Model file for the job. Use its own axes, mm. Give positions to 0.01 mm unless a question says otherwise; leave off trailing zeros.
```python
from build123d import *

# Parameters (mm, degrees)
BOX_W     = 300
BOX_H     = 100
BOX_DEPTH = 140


with BuildPart() as cubo:
    # Box → Box (new body)
    with BuildSketch(Plane(origin=(50, -50, -70), x_dir=(1, 0, 0), z_dir=(0, 0, 1))):
        with Locations((150, 50)):
            Rectangle(BOX_W, BOX_H)
    extrude(amount=BOX_DEPTH)


with BuildPart() as loft001:
    # Sketch003 → Loft001 section 0
    with BuildSketch(Plane(origin=(-5, 0, 0), x_dir=(1, 0, 0), z_dir=(0, 0, 1))):
        Polygon((300, 0), (299.703, 0.018), (298.818, 0.072), (297.342, 0.183), (295.287, 0.363), (292.659, 0.621), (289.467, 0.957), (285.723, 1.368), (281.445, 1.851), (276.648, 2.403), (271.353, 3.027), (265.578, 3.732), (259.344, 4.509), (252.681, 5.364), (245.613, 6.288), (238.167, 7.281), (230.373, 8.337), (222.264, 9.45), (213.867, 10.611), (205.218, 11.811), (196.353, 13.038), (187.305, 14.286), (178.107, 15.534), (168.801, 16.767), (159.42, 17.97), (150, 19.119), (140.583, 20.193), (131.199, 21.174), (121.893, 22.038), (112.698, 22.761), (103.647, 23.322), (94.782, 23.703), (86.133, 23.886), (77.736, 23.856), (69.627, 23.607), (61.833, 23.127), (54.387, 22.419), (47.319, 21.486), (40.656, 20.34), (34.422, 18.996), (28.647, 17.472), (23.352, 15.798), (18.555, 13.998), (14.277, 12.105), (10.533, 10.155), (7.341, 8.184), (4.713, 6.246), (2.658, 4.41), (1.182, 2.745), (0.297, 1.281), (0, 0), (0.297, -1.17), (1.182, -2.301), (2.658, -3.432), (4.713, -4.548), (7.341, -5.607), (10.533, -6.576), (14.277, -7.443), (18.555, -8.208), (23.352, -8.877), (28.647, -9.459), (34.422, -9.969), (40.656, -10.41), (47.319, -10.797), (54.387, -11.133), (61.833, -11.427), (69.627, -11.682), (77.736, -11.901), (86.133, -12.084), (94.782, -12.225), (103.647, -12.327), (112.698, -12.381), (121.893, -12.384), (131.199, -12.327), (140.583, -12.207), (150, -12.018), (159.42, -11.757), (168.801, -11.418), (178.107, -11.007), (187.305, -10.524), (196.353, -9.972), (205.218, -9.357), (213.867, -8.691), (222.264, -7.983), (230.373, -7.248), (238.167, -6.492), (245.613, -5.736), (252.681, -4.989), (259.344, -4.269), (265.578, -3.582), (271.353, -2.94), (276.648, -2.355), (281.445, -1.827), (285.723, -1.359), (289.467, -0.954), (292.659, -0.618), (295.287, -0.363), (297.342, -0.183), (298.818, -0.072), (299.703, -0.018), align=None)
    # Sketch004 → Loft001 section 1
    with BuildSketch(Plane(origin=(25, 0, 70), x_dir=(1, 0, 0), z_dir=(0, 0, 1))):
        Polygon((300, 0), (299.703, 0.018), (298.818, 0.072), (297.342, 0.183), (295.287, 0.363), (292.659, 0.621), (289.467, 0.957), (285.723, 1.368), (281.445, 1.851), (276.648, 2.403), (271.353, 3.027), (265.578, 3.732), (259.344, 4.509), (252.681, 5.364), (245.613, 6.288), (238.167, 7.281), (230.373, 8.337), (222.264, 9.45), (213.867, 10.611), (205.218, 11.811), (196.353, 13.038), (187.305, 14.286), (178.107, 15.534), (168.801, 16.767), (159.42, 17.97), (150, 19.119), (140.583, 20.193), (131.199, 21.174), (121.893, 22.038), (112.698, 22.761), (103.647, 23.322), (94.782, 23.703), (86.133, 23.886), (77.736, 23.856), (69.627, 23.607), (61.833, 23.127), (54.387, 22.419), (47.319, 21.486), (40.656, 20.34), (34.422, 18.996), (28.647, 17.472), (23.352, 15.798), (18.555, 13.998), (14.277, 12.105), (10.533, 10.155), (7.341, 8.184), (4.713, 6.246), (2.658, 4.41), (1.182, 2.745), (0.297, 1.281), (0, 0), (0.297, -1.17), (1.182, -2.301), (2.658, -3.432), (4.713, -4.548), (7.341, -5.607), (10.533, -6.576), (14.277, -7.443), (18.555, -8.208), (23.352, -8.877), (28.647, -9.459), (34.422, -9.969), (40.656, -10.41), (47.319, -10.797), (54.387, -11.133), (61.833, -11.427), (69.627, -11.682), (77.736, -11.901), (86.133, -12.084), (94.782, -12.225), (103.647, -12.327), (112.698, -12.381), (121.893, -12.384), (131.199, -12.327), (140.583, -12.207), (150, -12.018), (159.42, -11.757), (168.801, -11.418), (178.107, -11.007), (187.305, -10.524), (196.353, -9.972), (205.218, -9.357), (213.867, -8.691), (222.264, -7.983), (230.373, -7.248), (238.167, -6.492), (245.613, -5.736), (252.681, -4.989), (259.344, -4.269), (265.578, -3.582), (271.353, -2.94), (276.648, -2.355), (281.445, -1.827), (285.723, -1.359), (289.467, -0.954), (292.659, -0.618), (295.287, -0.363), (297.342, -0.183), (298.818, -0.072), (299.703, -0.018), align=None)
    loft()


with BuildPart() as cut:
    # Part__Mirroring001: instance of Loft001
    add(loft001.part.mirror(Plane(origin=(0, 0, 0), x_dir=(0, 1, 0), z_dir=(0, 0, 1))))

    # Fusion: union Loft001
    add(loft001.part)

    # Cut: cut Cubo
    add(cubo.part, mode=Mode.SUBTRACT)


solid = cut.part
```
1. Pull direction Z, two halves, no side cores. Call faces 1 (the flat face through (40, 1, -70)), 2 (the flat face through (40, 1, 70)), 3 (the flat face through (50, 5, -1)): +Z half, -Z half, draft (parallel to the pull), parting line (faces both ways), or undercut.
Calculated:
face 1: -Z half
face 2: +Z half
face 3: draft
2. Probe probe 1 along X at (y, z) = (11, -5); probe 2 along X at (y, z) = (12, 0); probe 3 along Y at (x, z) = (38, 28). List the from-to ranges inside material, lowest first.
Calculated:
probe 1: x = 9.3 to 50
probe 2: x = 9.08 to 50
probe 3: y = -9.67 to 18.09
3. Pin check, flat tips, straight feed: P1, Ø2, axis at x = 41.5, z = 20.5, coming from the -Y side; P2, Ø2, axis at y = 4, z = 46.5, coming from the -X side; P3, Ø2, axis at y = -4, z = 46.5, coming from the -X side. Stop position of each tip, or through.
Calculated:
P1: stops at y = -10.28
P2: stops at x = 16.24
P3: stops at x = 16.95
